Source: CAD feature listing. Evaluate the final solid. Frame: model axes, mm. A direction names the side the tool comes from. Give positions to 0.01 mm unless a question says otherwise; leave off trailing zeros. Write each loop counter-clockwise with the first axis right and the second up, starting at its lowest first coordinate (ties: lowest second). Pieces come first, ordered by that corner, then holes. Notation, with made-up numbers: M 35.5,27 L 70.5,27 A28 ccw 70.5,57 Z; hole C -18.75,12.5 d1. An arc over 180 degrees is marked long. Answer as a JSON object with one key per item and string values. Group by question number.
Autodesk Inventor part; units mm, degrees
ref_plane "Work Plane1" through (-40, 0, 0) normal (0.7071, -0.7071, 0) x (0, 0, 1)
ref_plane "YZ Plane" through (0, 0, 0) normal (1, 0, 0) x (0, 1, 0)
ref_plane "XZ Plane" through (0, 0, 0) normal (0, 1, 0) x (-1, 0, 0)
sketch "Sketch1" plane through (0, 0, 0) normal (0, 1, 0) x (-1, 0, 0)
  line L0 (0, 0) -> (40, 0)
  line L1 (40, 0) -> (40, -40)
  line L2 (40, -40) -> (0, -40)
  line L3 (0, -40) -> (0, 0)
  dimension "d0" = 40
  dimension "d1" = 40
extrude "Extrusion1" add sketch "Sketch1" along normal blind 6
fillet "Fillet1" radius 5 1 edges at (-40, 0, -20)
fillet "Fillet2" radius 5 1 edges at (0, 6, -20)
sketch "Sketch2" plane through (0, 6, 0) normal (0, 1, 0) x (1, 0, 0)
  line L0 (-5, 40) -> (-5, 0)
  line L1 (-35, 40) -> (-35, 0)
  circle A0 centre (-20, 10) radius 2.75
  line L2 (-40, 0) -> (-5, 0)
  circle A1 centre (-20, 30) radius 2.75
  point P0 (0, 0)
  dimension "d6" = 5.5
  dimension "d7" = 30
  dimension "d8" = 40
  dimension "d9" = 10
  dimension "d10" = 15
  dimension "d22" = 20
ref_plane "Work Plane1" through (-40, 0, 0) normal (0.7071, -0.7071, 0) x (0, 0, 1)
mirror "Mirror1" about plane through (-40, 0, 0) normal (0.7071, -0.7071, 0) of "Extrusion1", "Fillet2"
fillet "Fillet3" radius 5 1 edges at (-34, 6, -20)
extrude "Extrusion4" cut sketch "Sketch2" against normal blind 10
mirror "Mirror2" about plane through (-40, 0, 0) normal (0.7071, -0.7071, 0) of "Extrusion4"
equation "\"d9\" = 0.25 * d8"
equation "\"d10\" = 0.5 * d7"
properties part number "L_Fixer2" material "Steel, Carbon"
(1) Section A-A, the plane z = -10. Return loops of the section in (x, y).
(2) Section D-D, the plane z = -20.5. Return loops of the section in (x, y), plus the area to 3 significant figures.
(3) Contact query for flat-ended pins moving along their axis: pin 1 Ø6 at (x, z) = (-35, -12) entering from +Y; pin 2 Ø1 at (y, z) = (34.5, -29.5) entering from +X; pin 3 Ø6.5 at (x, z) = (-20, -30) entering from +Y; pin 4 Ø4.5 at (x, z) = (-20, -10) entering from +Y. Output: stop coordinate, or through.
(4) Section C-C, the plane x = -20. Return loops of the section in (y, z).
(5) Pull-direction query (X, two-part tool) for faces 1 (the flat face through (-17, 6, -20)), 2 (the cylindrical face through (-22.747, 3.042, -10.121)), 3 (the cylindrical face through (-35, 38, -20)); classes: pulls with the +X half, pulls with the -X half, needs draft (parallel to the pull), parting line crosses it, or undercut.
(6) Ray query, L1, parallel to Z at x = -36, y = 20; L2, parallel to X at y = 27, z = -4; L3, parallel to Y at x = -26.5, z = -18.5. Return the intervals inside material, ascending. Write a range as [from, to].
(7) Section B-B, the plane y = 20. Return loops of the section in (x, z).
(8) Access query for faces 4 (the flat face through (-20, 0, -20)), 5 (the flat face through (-34, 23, -20)). Directions: +Z, -Z, +X, -X, +Y, -Y. A direction counts if a zero-diameter tool reaches every point of the face in a straight line with its end or side. Return the directions, or none.
Reported:
{
 "1": {"outline": "M -40,0 L -22.75,0 L -22.75,6 L -29,6 A5 cw -34,11 L -34,17.25 L -40,17.25 Z; M -40,22.75 L -34,22.75 L -34,35 A5 ccw -39,40 L -40,40 Z; M -17.25,0 L 0,0 L 0,1 A5 ccw -5,6 L -17.25,6 Z"},
 "2": {"outline": "M -40,0 L 0,0 L 0,1 A5 ccw -5,6 L -29,6 A5 cw -34,11 L -34,35 A5 ccw -39,40 L -40,40 Z", "area": "439 mm2"},
 "3": {"pin 1": "stops at y = 39.9", "pin 2": "stops at x = -34", "pin 3": "stops at y = 6", "pin 4": "passes through"},
 "4": {"outline": "M 0,-40 L 6,-40 L 6,-32.75 L 0,-32.75 Z; M 0,-27.25 L 6,-27.25 L 6,-12.75 L 0,-12.75 Z; M 0,-7.25 L 6,-7.25 L 6,0 L 0,0 Z"},
 "5": {"face 1": "needs draft", "face 2": "undercut", "face 3": "pulls with the +X half"},
 "6": {"L1": "z = [-40, -32.75], [-27.25, -12.75], [-7.25, 0]", "L2": "x = [-40, -34]", "L3": "y = [0, 6]"},
 "7": {"outline": "M -40,-40 L -34,-40 L -34,-32.75 L -40,-32.75 Z; M -40,-27.25 L -34,-27.25 L -34,-12.75 L -40,-12.75 Z; M -40,-7.25 L -34,-7.25 L -34,0 L -40,0 Z"},
 "8": {"face 4": "+Z, -Z, +X, -X, -Y", "face 5": "+Z, -Z, +X, +Y"}
}
